Work out the finished part from the listing and answer in its coordinate system (mm). A direction names the side the tool comes from. Coordinates: 2 decimals unless noted, no trailing zeros. Write each loop counter-clockwise with the first axis right and the second up, starting at its lowest first coordinate (ties: lowest second). Pieces come first, ordered by that corner, then holes. Notation, with made-up numbers: (15.25, -2) - (35.25, -2) arc R8 ccw to (35.25, 11) - close; hole circle Ø6 at (-30, 6). An arc over 180 degrees is marked (long way). Answer as a JSON object with one key per item and string values. Group by question number.
from build123d import *

# Parameters (mm, degrees)
SZKIC1_W                        = 8
SZKIC1_H                        = 40
WYTNIJ_WYCI_GNI_CIE1_DEPTH      = 22
WYTNIJ_WYCI_GNI_CIE1_DEPTH_BACK = 22
SZKIC3_R                        = 16
WYTNIJ_WYCI_GNI_CIE2_DEPTH      = 9
WYTNIJ_WYCI_GNI_CIE2_DEPTH_BACK = 9
SFAZOWANIE1_SIZE                = 2


with BuildPart() as part:
    # Szkic1 → Obrót1 (revolve)
    with BuildSketch(Plane(origin=(0, 0, 0), x_dir=(1, 0, 0), z_dir=(0, 1, 0))):
        with BuildLine():
            Line((0, 21), (0, -26))
            Line((0, -26), (8, -26))
            Line((8, -26), (17.525976473, -11.568930316))
            ThreePointArc((17.525976473, -11.568930316), (18.492532772, 9.951192475), (0, 21))
        make_face()
        with Locations((4, -46)):
            Rectangle(SZKIC1_W, SZKIC1_H)
    revolve(axis=Axis((0, 0, -26.043516498), (0, 0, 1)))

    # Szkic2 → Wytnij-wyciągnięcie1 (cut, two sides)
    with BuildSketch(Plane(origin=(0, 0, 0), x_dir=(0, 0, -1), z_dir=(1, 0, 0))) as wytnij_wyci_gni_cie1_sk:
        with BuildLine():
            Line((-26, 8), (19.416487839, 8))
            ThreePointArc((19.416487839, 8), (6.171069333, 20.072815031), (-11.568930316, 17.525976473))
            Line((-11.568930316, 17.525976473), (-26, 8))
        make_face()
        with BuildLine():
            Line((-26, -8), (19.416487839, -8))
            ThreePointArc((19.416487839, -8), (6.171069333, -20.072815031), (-11.568930316, -17.525976473))
            Line((-11.568930316, -17.525976473), (-26, -8))
        make_face()
    extrude(amount=WYTNIJ_WYCI_GNI_CIE1_DEPTH, mode=Mode.SUBTRACT)
    extrude(wytnij_wyci_gni_cie1_sk.sketch, amount=-WYTNIJ_WYCI_GNI_CIE1_DEPTH_BACK, mode=Mode.SUBTRACT)

    # Szkic3 → Wytnij-wyciągnięcie2 (cut, two sides)
    with BuildSketch(Plane(origin=(0, 0, 0), x_dir=(1, 0, 0), z_dir=(0, 1, 0))) as wytnij_wyci_gni_cie2_sk:
        Circle(SZKIC3_R)
    extrude(amount=WYTNIJ_WYCI_GNI_CIE2_DEPTH, mode=Mode.SUBTRACT)
    extrude(wytnij_wyci_gni_cie2_sk.sketch, amount=-WYTNIJ_WYCI_GNI_CIE2_DEPTH_BACK, mode=Mode.SUBTRACT)

    # Sfazowanie1
    sfazowanie1_edges = [part.edges().sort_by_distance(p)[0] for p in [
        (-8, 0, 66),
    ]]
    chamfer(sfazowanie1_edges, length=SFAZOWANIE1_SIZE)


solid = part.part
Q1. Section C-C on z = 30 is taken. Determine the outline of the cut face in (x, y), plus the area to 3 significant figures.
Q2. Consider L1, parallel to X at y = 0.25, z = 0; L2, parallel to X at y = 0.5, z = 27; L3, parallel to X at y = 2.75, z = 14.5. Determine where each line is inside the solid, lowest interval first. Write a range as from..to.
Q3. Section A-A on z = 0 is taken. Determine the outline of the cut face in (x, y), plus the area to 3 significant figures.
Q4. Flat-ended cylindrical pins translate along their axes: pin 1 Ø1 at (x, y) = (6.5, -2) entering from +Z; pin 2 Ø3 at (y, z) = (-5.5, 54) entering from -X; pin 3 Ø5 at (x, y) = (10.5, 2.5) entering from +Z. Find the tip coordinate at first contact, or state that the pin passes through.
Q5. A tool of negligible diameter and unlimited length cuts with its end or side. For faces 5 (the face through (-1.73, -7.81, 44.73)), 6 (the face through (0, 0, 66)), from which of +Z, -Z, +X, -X, +Y, -Y can it reach the whole face along a straight path? Write none if from no direction.
Q6. Section B-B on y = 0 is taken. Determine the outline of the cut face in (x, z), plus the area to 3 significant figures.
Q7. Section D-D on z = 17 is taken. Determine the outline of the cut face in (x, y), plus the area to 3 significant figures.
Q8. For a pull along X with two mould halves and no side action, classify faces 1 (the face through (6, -8, 15)), 2 (the face through (-4.861, -3.727, 65.875)), 3 (the face through (11.768, -0.259, 20.287)), 4 (the face through (-3.47, 0.11, 15.62)) as +X half, -X half, draft (parallel to the pull), parting line (faces both ways), or undercut.
Numbers:
{
 "1": {"outline": "circle Ø16 at (0, 0)", "area": "201 mm²"},
 "2": {"L1": "x = -21..-16, 16..21", "L2": "x = -7.98..7.98", "L3": "x = -15.35..-6.76, 6.76..15.35"},
 "3": {"outline": "(-19.42, -8) - (-16, -8) - (-16, 8) - (-19.42, 8) arc R21 ccw to start; (16, -8) - (19.42, -8) arc R21 ccw to (19.42, 8) - (16, 8) - close", "area": "143 mm²"},
 "4": {"pin 1": "stops at z = 65.7", "pin 2": "stops at x = -6.93", "pin 3": "stops at z = 25.56"},
 "5": {"face 5": "+Z", "face 6": "+Z, +X, -X, +Y, -Y"},
 "6": {"outline": "(-17.53, 11.57) arc R21 ccw (long way) to (17.53, 11.57) - (8, 26) - (8, 64) - (6, 66) - (-6, 66) - (-8, 64) - (-8, 26) - close; hole circle Ø32 at (0, 0)", "area": "1,350 mm²"},
 "7": {"outline": "(-11.42, -8) - (11.42, -8) arc R13.94 ccw to (11.42, 8) - (-11.42, 8) arc R13.94 ccw to start", "area": "420 mm²"},
 "8": {"face 1": "draft", "face 2": "parting line", "face 3": "+X half", "face 4": "undercut"}
}
